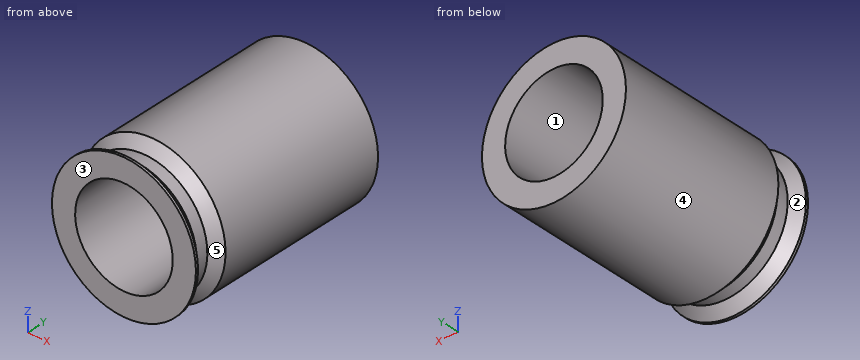
from build123d import *

# Parameters (mm, degrees)
SKETCH_1_R      = 2.95
SKETCH_1_R_2    = 2
EXTRUDE_1_DEPTH = 4.3
SKETCH_2_W      = 0.4
SKETCH_2_H      = 0.5
CHAMFER_1_SIZE  = 0.4


with BuildPart() as part:
    # 草图1 → 凸台-拉伸1 (new, symmetric)
    with BuildSketch(Plane(origin=(0, 0, 0), x_dir=(1, 0, 0), z_dir=(0, 1, 0))):
        with Locations(Location((0, 0, 0), (0, 0, 90))):
            Circle(SKETCH_1_R)
        with Locations(Location((0, 0, 0), (0, 0, 90))):
            Circle(SKETCH_1_R_2, mode=Mode.SUBTRACT)
    extrude(amount=EXTRUDE_1_DEPTH, both=True)

    # 草图2 → 切除-旋转1 (revolve, cut)
    with BuildSketch(Plane(origin=(0, 0, 0), x_dir=(0, 0, -1), z_dir=(1, 0, 0)), mode=Mode.PRIVATE) as cut_revolve_1_sk:
        with Locations((-2.75, -3.55)):
            Rectangle(SKETCH_2_W, SKETCH_2_H)
    revolve(cut_revolve_1_sk.sketch.rotate(Axis((0, -1000, 0), (0, 1, 0)), 180), axis=Axis((0, -1000, 0), (0, 1, 0)), mode=Mode.SUBTRACT)

    # 倒角1
    chamfer_1_edges = [part.edges().sort_by_distance(p)[0] for p in [
        (0, -3.3, 2.95),
        (0, -3.8, 2.95),
    ]]
    chamfer(chamfer_1_edges, length=CHAMFER_1_SIZE - 0.0001)  # a hair under: the kernel refuses the full size


solid = part.part
Read the model definition and answer for the solid it produces. Units are mm, in the model's axes. Face numbers are marked on the shaded views. A direction names the side the tool comes from. Round coordinates to 2 decimals unless told otherwise and drop trailing zeros. Order: outer loops, then holes, each group sorted by start corner. A loop starts at its lowest first (then second) coordinate and runs counter-clockwise, first axis right, second up.
1) Straight lines are drawn through the part: L1, parallel to X at y = 0.25, z = 0; L2, parallel to Z at x = -0.1, y = -3.5; L3, parallel to Z at x = 1.55, y = 3.5. For each, find the intervals that lie inside material, in ascending order.
2) The mould has two halves that part along Z. Classify the marked faces 1, 2 and 3: released by +Z, released by -Z, zero draft, split by the parting line, or undercut.
3) For the marked faces 4 and 5, determine the directions among +Z, -Z, +X, -X, +Y, -Y from which every point of the face is accessible in a straight line to the end or side of a thin tool.
4) The part is cut by section C-C on y = 2. Write down the section's boundary in (x, z), plus the area to 3 significant figures.
5) Flat-ended cylindrical pins translate along their axes: pin 1 (3 mm diameter, centred on x = 0, z = 0, fed in from +Y); pin 2 (1.5 mm diameter, centred on x = -1, y = 1.5, fed in from -Z). Find the tip coordinate at first contact, or state that the pin passes through.
Resolved:
1. L1: x = -2.95 to -2, 2 to 2.95
1. L2: z = -2.55 to -2, 2 to 2.55
1. L3: z = -2.51 to -1.26, 1.26 to 2.51
2. face 1: undercut
2. face 2: split by the parting line
2. face 3: zero draft
3. face 4: +Y, -Y
3. face 5: none
4. outline: circle Ø5.9 at (0, 0); hole circle Ø4 at (0, 0)
4. area: 14.8 mm2
5. pin 1: passes through
5. pin 2: stops at z = -2.94
